Study the drawing (mm; zero at the part's minimum x, y, z) and answer. A direction names the side the tool comes from. Round coordinates to 2 decimals unless told otherwise and drop trailing zeros. Loops run counter-clockwise (first coordinate to the right, second up) from the corner with the lowest first, then second, coordinate; pieces in that order, holes last. Notation, with made-up numbers: (47, 17) -> (77, 17) arc R19 ccw to (77, 32) -> close; hole circle Ø9 at (64, 65.25). An arc over 180 degrees is marked (long way). Answer in a Markdown table with one row per item. Add a question column.
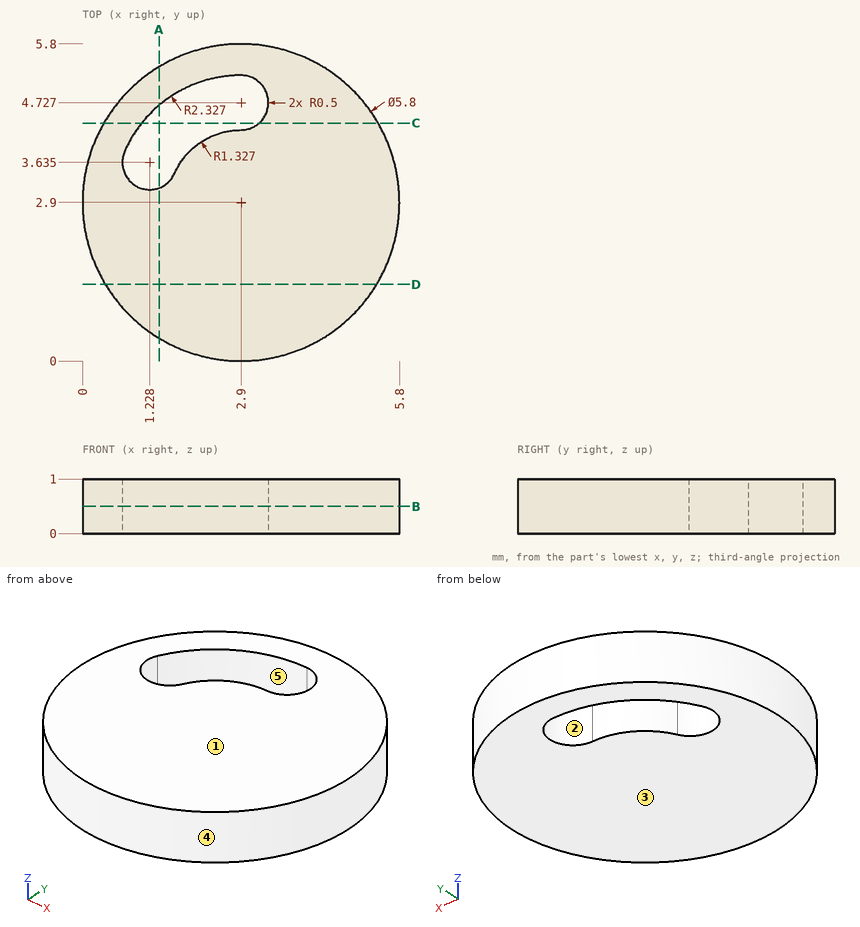
Item 1: Section D-D, the plane y = 1.4 is taken. Write down the section's boundary in (x, z).
Item 2: Section A-A, the plane x = 1.4 is taken. Write down the section's boundary in (y, z) (1 decimal).
Item 3: For the marked faces 1 and 2, determine the directions among +Z, -Z, +X, -X, +Y, -Y from which every point of the face is accessible in a straight line to the end or side of a thin tool.
Item 4: Section C-C, the plane y = 4.35 is taken. Write down the section's boundary in (x, z).
Item 5: Consider L1, parallel to X at y = 4.55, z = 0.7 (1 decimal); L2, parallel to Y at x = 2.1, z = 0.15 (1 decimal); L3, parallel to Y at x = 2.8, z = 0.5 (1 decimal). Determine where each line is inside the solid, lowest interval first. Write a range as from..to.
Item 6: The mould has two halves that part along Y. Classify the marked faces 3, 4 and 5: +Y half, -Y half, draft (parallel to the pull), parting line (faces both ways), or undercut.
Item 7: Section B-B, the plane z = 0.5 is taken. Write down the section's boundary in (x, y) (1 decimal), and give its area (3 significant figures).
Here are the results:
| question | item | result |
|---|---|---|
| 1 | outline | (0.42, 0) -> (5.38, 0) -> (5.38, 1) -> (0.42, 1) -> close |
| 2 | outline | (0.4, 0) -> (3.2, 0) -> (3.2, 1) -> (0.4, 1) -> close; (4.7, 0) -> (5.4, 0) -> (5.4, 1) -> (4.7, 1) -> close |
| 3 | face 1 | +Z, +X, -X, +Y, -Y |
| 3 | face 2 | +Z, -Z |
| 4 | outline | (0.39, 0) -> (1.08, 0) -> (1.08, 1) -> (0.39, 1) -> close; (3.23, 0) -> (5.41, 0) -> (5.41, 1) -> (3.23, 1) -> close |
| 5 | L1 | x = 0.5..1.3, 3.4..5.3 |
| 5 | L2 | y = 0.1..4, 5.1..5.7 |
| 5 | L3 | y = 0..4.2, 5.2..5.8 |
| 6 | face 3 | draft |
| 6 | face 4 | parting line |
| 6 | face 5 | undercut |
| 7 | outline | circle Ø5.8 at (2.9, 2.9); hole (0.8, 3.8) arc R0.5 ccw to (1.7, 3.4) arc R1.3 cw to (2.9, 4.2) arc R0.5 ccw to (2.9, 5.2) arc R2.3 ccw to start |
| 7 | area | 23.5 mm² |
